Source: CAD feature listing. Evaluate the final solid. Frame: model axes, mm. Face numbers are marked on the shaded views. A direction names the side the tool comes from. Give positions to 0.01 mm unless a question says otherwise; leave off trailing zeros. Order: outer loops, then holes, each group sorted by start corner. A loop starts at its lowest first (then second) coordinate and runs counter-clockwise, first axis right, second up. Notation, with made-up numbers: (50, 68) - (85, 68) arc R15 cw to (85, 91) - close; hole circle Ø2 at (2, -10). An arc over 180 degrees is marked (long way). Answer as CSV lines item,"result".
```python
from build123d import *

# Parameters (mm, degrees)
EXTRUDE_9_DEPTH     = 237
CUT_EXTRUDE_3_DEPTH = 78
SKETCH_12_W         = 13
SKETCH_12_H         = 22
CUT_EXTRUDE_5_DEPTH = 110
SKETCH_13_R         = 11
CUT_EXTRUDE_6_DEPTH = 13
SKETCH_14_W         = 33
SKETCH_14_H         = 63.965487913
CUT_EXTRUDE_9_DEPTH = 19
EXTRUDE_START       = 33
EXTRUDE_11_DEPTH    = 33


with BuildPart() as part:
    # 草图1 → 凸台-拉伸9 (new body)
    with BuildSketch(Plane(origin=(0, 0, 0), x_dir=(0, 0, -1), z_dir=(1, 0, 0))):
        with BuildLine():
            Line((0, 172), (0, 114.575))
            ThreePointArc((0, 114.575), (-28.575, 86), (0, 57.425))
            Line((0, 57.425), (0, 0))
            Line((0, 0), (-13, 0))
            Line((-13, 0), (-86, 42.146569651))
            Line((-86, 42.146569651), (-86, 86))
            ThreePointArc((-86, 86), (-60.811183182, 146.811183182), (0, 172))
        make_face()
    extrude(amount=-EXTRUDE_9_DEPTH)

    # 草图1<13> → 切除-拉伸3 (cut)
    with BuildSketch(Plane(origin=(0, 0, 0), x_dir=(0, 0, -1), z_dir=(1, 0, 0))):
        with BuildLine():
            Line((0, 114.575), (0, 130.45))
            ThreePointArc((0, 130.45), (-44.45, 86), (0, 41.55))
            Line((0, 41.55), (0, 57.425))
            ThreePointArc((0, 57.425), (-28.575, 86), (0, 114.575))
        make_face()
    extrude(amount=-CUT_EXTRUDE_3_DEPTH, mode=Mode.SUBTRACT)

    # 草图12 → 切除-拉伸5 (cut)
    with BuildSketch(Plane.ZY.offset(237)):
        with Locations((6.5, 26)):
            Rectangle(SKETCH_12_W, SKETCH_12_H)
    extrude(amount=-CUT_EXTRUDE_5_DEPTH, mode=Mode.SUBTRACT)

    # 草图13 → 切除-拉伸6 (cut)
    with BuildSketch(Plane(origin=(0, 0, 0), x_dir=(-1, 0, 0), z_dir=(0, 0, -1))):
        with Locations((127, 26)):
            Circle(SKETCH_13_R)
    extrude(amount=-CUT_EXTRUDE_6_DEPTH, mode=Mode.SUBTRACT)

    # 草图14 → 切除-拉伸9 (cut)
    with BuildSketch(Plane(origin=(0, 0, 0), x_dir=(-1, 0, 0), z_dir=(0, 0, -1))):
        with Locations((182.5, 140.017256043)):
            Rectangle(SKETCH_14_W, SKETCH_14_H)
    extrude(amount=-CUT_EXTRUDE_9_DEPTH, mode=Mode.SUBTRACT)

    # 草图10 → 凸台-拉伸11 (add)
    with BuildSketch(Plane(origin=(0, 0, 0), x_dir=(0, 0, -1), z_dir=(1, 0, 0)).offset(EXTRUDE_START)):
        with BuildLine():
            Line((-84.813857215, 100.234100753), (-65.430668922, 85.090294344))
            Line((-65.430668922, 85.090294344), (-14.946427946, 149.707176139))
            Line((-14.946427946, 149.707176139), (-34.329616239, 164.850982549))
            ThreePointArc((-34.329616239, 164.850982549), (-67.76892481, 138.946886878), (-84.813857215, 100.234100753))
        make_face()
    extrude(amount=-EXTRUDE_11_DEPTH)


solid = part.part
```
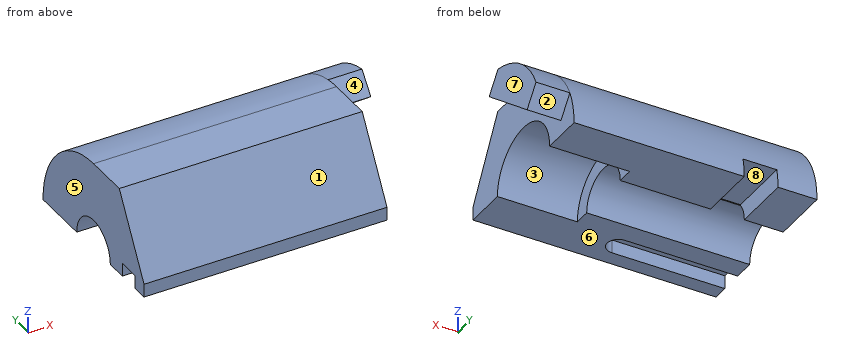
(1) Cut plane D-D (x = 12). Return loops of the section in (y, z), then the cut area to 3 significant figures.
Completed:
outline,"(85.09, 65.43) - (149.71, 14.95) - (164.85, 34.33) arc R86 ccw to (100.23, 84.81) - close"
area,"2,590 mm²"
(2) Ray query, line 1 (X direction, y = 155, z = 5); line 2 (X direction, y = 119.5, z = 23.5); line 3 (Y direction, x = -123, z = 5). Return the intervals inside material, ascending. Write a range as from..to.
Completed:
line 1,"-237..-199, -166..0"
line 2,"-237..-78"
line 3,"0..15.75, 36.25..57.87, 114.13..171.85"
(3) Mould query, pull axis X, two halves, no side actions, for the marked faces 5, 6, 7 and 8. Classes: released by +X, released by -X, zero draft, split by the parting line, or undercut.
Completed:
face 5,"released by -X"
face 6,"zero draft"
face 7,"released by +X"
face 8,"undercut"
(4) Cut plane B-B (z = 73). Return loops of the section in (x, y), then the cut area to 3 significant figures.
Completed:
outline,"(-237, 34.64) - (0, 34.64) - (0, 91) - (33, 91) - (33, 131.46) - (-237, 131.46) - close"
area,"24,300 mm²"
(5) Access query for the marked faces 1, 2, 3 and 4. Directions: +Z, -Z, +X, -X, +Y, -Y. A direction counts if a zero-diameter tool reaches every point of the face in a straight line with its end or side. Return the directions, or none.
Completed:
face 1,"+Z, +X, -X, -Y"
face 2,"-Z, +X, +Y"
face 3,"-Z, +X"
face 4,"+Z, +X, -Y"
(6) Contact query for flat-ended pins moving along their axis: pin 1 (0.6 mm diameter, centred on x = -179.5, z = 18.5, fed in from +Y); pin 2 (15 mm diameter, centred on y = 126, z = 10, fed in from +X); pin 3 (4 mm diameter, centred on x = -62.5, z = 52.5, fed in from -Y); pin 4 (14.5 mm diameter, centred on x = -172, z = 7, fed in from -Y). Output: stop coordinate, or through.
Completed:
pin 1,"y = 108.03"
pin 2,"x = 0"
pin 3,"y = 21.65"
pin 4,"y = 0"
(7) Cut plane C-C (y = 26). Return loops of the section in (x, z).
Completed:
outline,"(-237, 13) - (-116, 13) - (-116, 0) - (0, 0) - (0, 58.03) - (-237, 58.03) - close"
(8) Cut plane A-A (x = -100.5). Return loops of the section in (y, z) (3 decimals).
Completed:
outline,"(0, 0) - (57.425, 0) arc R28.575 cw to (114.575, 0) - (172, 0) arc R86 ccw to (86, 86) - (42.147, 86) - (0, 13) - close"
